Design review of the part shown in the three views and the two pictorial views. Dimensions are in mm from the part's minimum x, y and z. Give positions to 0.01 mm unless a question says otherwise; leave off trailing zeros. Order: outer loops, then holes, each group sorted by start corner. A loop starts at its lowest first (then second) coordinate and runs counter-clockwise, first axis right, second up. Notation, with made-up numbers: M 52,-13 L 66,-13 A12 ccw 66,1 Z; hole C 84,-10.75 d10. An arc over 180 degrees is marked long. Answer as a JSON object with one key per item and string values.
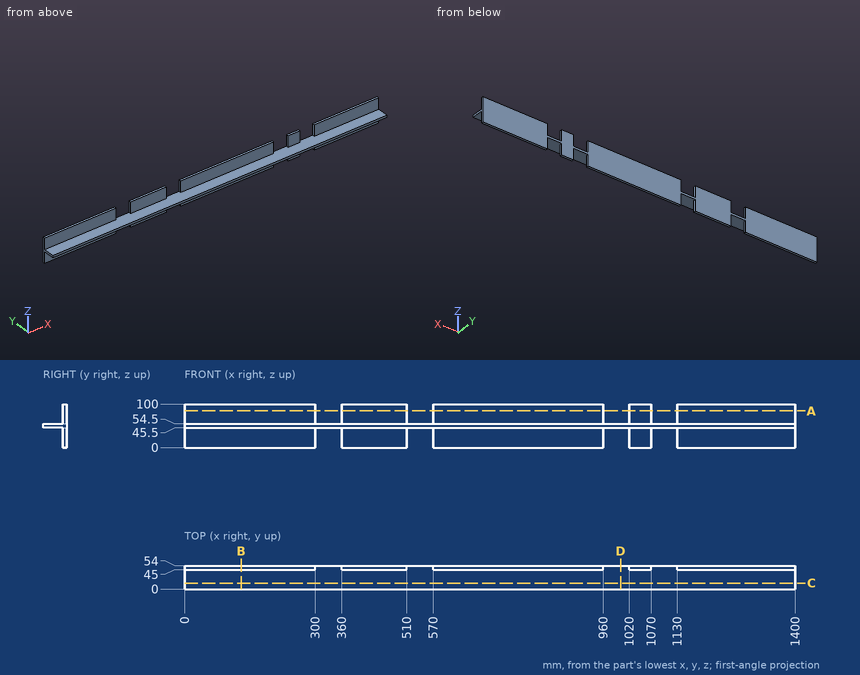
(1) We need section B-B (x = 129.5). Write out the cut boundary in (y, z).
Checked values:
{"outline": "M 0,45.5 L 45,45.5 L 45,0 L 54,0 L 54,100 L 45,100 L 45,54.5 L 0,54.5 Z"}
(2) We need section C-C (y = 14). Write out the cut boundary in (x, z), plus the area to 3 significant figures.
Checked values:
{"outline": "M 0,45.5 L 1400,45.5 L 1400,54.5 L 0,54.5 Z", "area": "12,600 mm^2"}
(3) To check wall thickness, follow L1, parallel to Y at x = 169, z = 65.5; L2, parallel to Z at x = 690, y = 20. State the ranges of each line that lie inside material, in increasing order. Write a range as from..to.
Checked values:
{"L1": "y = 45..54", "L2": "z = 45.5..54.5"}
(4) We need section D-D (x = 1000). Write out the cut boundary in (y, z), plus the area to 3 significant figures.
Checked values:
{"outline": "M 0,45.5 L 54,45.5 L 54,54.5 L 0,54.5 Z", "area": "486 mm^2"}
(5) Insertion check: pin 1 (8 mm diameter, centred on x = 435.5, y = 18, fed in from +Z); pin 2 (23 mm diameter, centred on x = 841, z = 17.5, fed in from -Y). Each pin has a flat end and moves straight along its axis. Give the tip position at first contact, or say it passes through.
Checked values:
{"pin 1": "stops at z = 54.5", "pin 2": "stops at y = 45"}
(6) We need section A-A (z = 84.5). Write out the cut boundary in (x, y).
Checked values:
{"outline": "M 0,45 L 300,45 L 300,54 L 0,54 Z; M 360,45 L 510,45 L 510,54 L 360,54 Z; M 570,45 L 960,45 L 960,54 L 570,54 Z; M 1020,45 L 1070,45 L 1070,54 L 1020,54 Z; M 1130,45 L 1400,45 L 1400,54 L 1130,54 Z"}
